Check sheet for the modelled part. Datum: model origin and axes. Units: mm. A direction names the side the tool comes from. Coordinates: 2 decimals unless noted, no trailing zeros. Loops run counter-clockwise (first coordinate to the right, second up) from the corner with the lowest first, then second, coordinate; pieces in that order, holes last. Notation, with made-up numbers: (45.5, -5) -> (84.5, -5) arc R24 ccw to (84.5, 26) -> close; hole circle Ø6 at (37, 40.5). An arc over 180 degrees is marked (long way). Use CSV: the item, a comma, the result in double quotes. Start each with the question number.
1. Thickness scan on L1, parallel to Y at x = 4, z = 22.5; L2, parallel to Y at x = 5.5, z = 27. Record the ranges inside material, lowest first.
2. Sectioned sample at A-A, the plane x = -8.5. Record the cut outline in (y, z).
3. Set-up check for faces 5 (the face through (-3.1, 9, 20)), 6 (the face through (-9, -3.1, 20)), 7 (the face through (9, -3.1, 20)), 8 (the face through (-5, 8, 20)): record each of +Z, -Z, +X, -X, +Y, -Y from which the full face is reachable in a straight line by a thin tool's end or side.
4. Sectioned sample at B-B, the plane y = 0. Record the cut outline in (x, z).
5. Gauge pin test, flat ends, axial feed: pin 1 (2 mm diameter, centred on x = -1, z = 13.5, fed in from +Y); pin 2 (3.5 mm diameter, centred on y = 1, z = 15, fed in from +X); pin 3 (4.5 mm diameter, centred on y = -0.5, z = 12.5, fed in from -X); pin 4 (8 mm diameter, centred on x = -2.5, z = 11, fed in from +Y). Record the tip position at first contact, or that the pin passes through.
6. Release check for a two-part mould opening along Y. For faces 1 (the face through (7, -10, 20)), 2 (the face through (2, 2, 40)), 3 (the face through (5.92, -4.15, 19.72)), 4 (the face through (4.15, -5.92, 20.28)) record: pulls with the +Y half, pulls with the -Y half, needs draft (parallel to the pull), parting line crosses it, or undercut.
```python
from build123d import *

# Parameters (mm, degrees)
SKETCH_W        = 20
SKETCH_H        = 20
PAD_DEPTH       = 40
SKETCH001_R     = 2.5
POCKET_DEPTH    = 40.001
POCKET001_DEPTH = 40.001


with BuildPart() as part:
    # Sketch → Pad (new body)
    with BuildSketch(Plane.XY):
        Rectangle(SKETCH_W, SKETCH_H)
    extrude(amount=PAD_DEPTH)

    # Sketch001 (on Face6 of Pad) → Pocket (cut, through all)
    with BuildSketch(Plane.XY.offset(40)):
        Circle(SKETCH001_R)
        Polygon((-3.1, 10), (3.1, 10), (3.1, 8), (6.232233, 8), (2.132233, 3.9), (-2.132233, 3.9), (-6.232233, 8), (-3.1, 8), align=None)
        Polygon((-3.1, -8), (-6.232233, -8), (-2.132233, -3.9), (2.132233, -3.9), (6.232233, -8), (3.1, -8), (3.1, -10), (-3.1, -10), align=None)
    extrude(amount=-POCKET_DEPTH, mode=Mode.SUBTRACT)

    # Sketch002 (on Face2 of Pocket) → Pocket001 (cut, through all)
    with BuildSketch(Plane(origin=(0, 0, 0), x_dir=(1, 0, 0), z_dir=(0, 0, -1))):
        Polygon((-10, -3.1), (-8, -3.1), (-8, -6.232233), (-3.9, -2.132233), (-3.9, 2.132233), (-8, 6.232233), (-8, 3.1), (-10, 3.1), align=None)
        Polygon((3.9, -2.132233), (3.9, 2.132233), (8, 6.232233), (8, 3.1), (10, 3.1), (10, -3.1), (8, -3.1), (8, -6.232233), align=None)
    extrude(amount=-POCKET001_DEPTH, mode=Mode.SUBTRACT)


solid = part.part
```
Completed:
1,L1,"-10 to -8, -5.77 to -2.23, 2.23 to 5.77, 8 to 10"
1,L2,"-10 to -8, -7.27 to -3.73, 3.73 to 7.27, 8 to 10"
2,outline,"(-10, 0) -> (-3.1, 0) -> (-3.1, 40) -> (-10, 40) -> close; (3.1, 0) -> (10, 0) -> (10, 40) -> (3.1, 40) -> close"
3,face 5,"+Z, -Z, +Y"
3,face 6,"+Z, -Z, -X"
3,face 7,"+Z, -Z, +X"
3,face 8,"+Z, -Z"
4,outline,"(-3.9, 0) -> (-2.5, 0) -> (-2.5, 40) -> (-3.9, 40) -> close; (2.5, 0) -> (3.9, 0) -> (3.9, 40) -> (2.5, 40) -> close"
5,pin 1,"y = 3.9"
5,pin 2,"x = 4.52"
5,pin 3,"x = -4.52"
5,pin 4,"y = 10"
6,face 1,"pulls with the -Y half"
6,face 2,"needs draft"
6,face 3,"undercut"
6,face 4,"undercut"
